Job drawing, mm, ordinate dimensions from the low corner. One solid piece. A direction names the side the tool comes from. Round coordinates to 2 decimals unless told otherwise and drop trailing zeros. Write each loop counter-clockwise with the first axis right and the second up, starting at its lowest first coordinate (ties: lowest second). Pieces come first, ordered by that corner, then holes. Notation, with made-up numbers: (72.25, -36) -> (104.25, -36) arc R8 ccw to (104.25, -22) -> close; hole circle Ø4 at (68.5, -27.5). An arc over 180 degrees is marked (long way). Use CSV: the item, a comma, the result in double quotes. Start each with the question number.
(1) Which spindle directions (+Z, -Z, +X, -X, +Y, -Y) get a long thin tool onto all of the face, cutting with end or side? Do the marked faces 1 and 2. Say none if no direction does.
(2) Saw through at C-C (x = 10). Give the cut face in (y, z), plus the area to 3 significant figures.
(3) Two-plate mould, pull along Y, no slides. Class the marked faces 3, 4 and 5: released by +Y, released by -Y, zero draft, split by the parting line, or undercut.
(4) Probe line 1 (Y direction, x = 24, z = 24.55); line 2 (Z direction, x = 15, y = 32); line 3 (Y direction, x = 24, z = 12.5). List the from-to ranges inside material, lowest first. Write a range as [from, to].
(5) Saw through at A-A (x = 24). Give the cut face in (y, z), plus the area to 3 significant figures.
(6) Saw through at D-D (y = 10.5). Give the cut face in (x, z).
(7) Saw through at B-B (y = 25). Give the cut face in (x, z), plus the area to 3 significant figures.
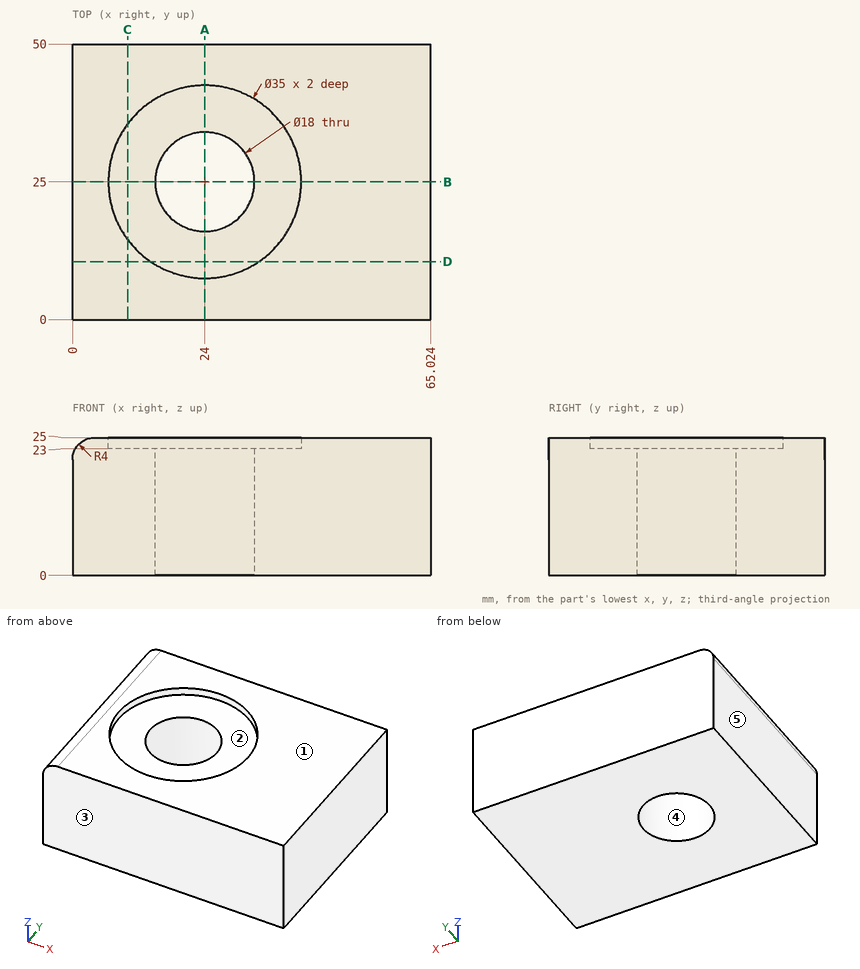
Answers:
1,face 1,"+Z, +X, -X, +Y, -Y"
1,face 2,"+Z"
2,outline,"(0, 0) -> (50, 0) -> (50, 25) -> (35.5, 25) -> (35.5, 23) -> (14.5, 23) -> (14.5, 25) -> (0, 25) -> close"
2,area,"1,210 mm²"
3,face 3,"released by -Y"
3,face 4,"undercut"
3,face 5,"zero draft"
4,line 1,"y = [0, 7.5], [42.5, 50]"
4,line 2,"z = [0, 23]"
4,line 3,"y = [0, 16], [34, 50]"
5,outline,"(0, 0) -> (16, 0) -> (16, 23) -> (7.5, 23) -> (7.5, 25) -> (0, 25) -> close; (34, 0) -> (50, 0) -> (50, 25) -> (42.5, 25) -> (42.5, 23) -> (34, 23) -> close"
5,area,"766 mm²"
6,outline,"(0, 0) -> (65.02, 0) -> (65.02, 25) -> (33.8, 25) -> (33.8, 23) -> (14.2, 23) -> (14.2, 25) -> (4, 25) arc R4 ccw to (0, 21) -> close"
7,outline,"(0, 0) -> (15, 0) -> (15, 23) -> (6.5, 23) -> (6.5, 25) -> (4, 25) arc R4 ccw to (0, 21) -> close; (33, 0) -> (65.02, 0) -> (65.02, 25) -> (41.5, 25) -> (41.5, 23) -> (33, 23) -> close"
7,area,"1,140 mm²"
